Can you work these out from the model? Positions are in its coordinate system, mm. A direction names the side the tool comes from. Round coordinates to 2 decimals unless told otherwise and drop trailing zeros. Loops run counter-clockwise (first coordinate to the right, second up) from the corner with the lowest first, then second, coordinate; pieces in that order, holes last.
from build123d import *

# Parameters (mm, degrees)
F1_DEPTH = 3


with BuildPart() as f1:
    # F0 (on Front) → F1 (new body)
    with BuildSketch(Plane.XZ):
        with BuildLine():
            ThreePointArc((0, 1.75), (1.75, 0), (0, -1.75))
            Line((0, -1.75), (-0.5, -1.75))
            ThreePointArc((-0.5, -1.75), (-1.394427, -1.538854), (-2.1, -0.95))
            ThreePointArc((-2.1, -0.95), (-6.124265, -1.312868), (-4, -4.75))
            Line((-4, -4.75), (0, -4.75))
            ThreePointArc((0, -4.75), (4.75, 0), (0, 4.75))
            Line((0, 4.75), (-20, 4.75))
            ThreePointArc((-20, 4.75), (-24.75, 0), (-20, -4.75))
            Line((-20, -4.75), (-16, -4.75))
            ThreePointArc((-16, -4.75), (-13.883666, -1.297152), (-17.920914, -0.978321))
            ThreePointArc((-17.920914, -0.978321), (-18.804769, -1.662707), (-19.917848, -1.765869))
            Line((-19.917848, -1.765869), (-20, -1.75))
            ThreePointArc((-20, -1.75), (-21.75, 0), (-20, 1.75))
            Line((-20, 1.75), (0, 1.75))
        make_face()
    extrude(amount=F1_DEPTH)


solid = f1.part
(1) If we section it at A-A, the plane x = 1.25: List the corners of the cut face in (y, z) for me, then the cut area to 3 significant figures.
Worked answers:
outline: (-3, -4.58) - (0, -4.58) - (0, -1.22) - (-3, -1.22) - close; (-3, 1.22) - (0, 1.22) - (0, 4.58) - (-3, 4.58) - close
area: 20.1 mm2
(2) For faces 1 (the flat face through (-10, -3, 2)), 2 (the cylindrical face through (-21.75, -1.48, -0.04)), which set-ups out of +Z, -Z, +X, -X, +Y, -Y let a thin tool reach every point of the face, with its end or its side?
Worked answers:
face 1: +Z, -Z, +X, -X, -Y
face 2: +Y, -Y
(3) If we section it at B-B, the plane z = -3.75: List the corners of the cut face in (x, y) for me.
Worked answers:
outline: (-22.92, -3) - (-14.06, -3) - (-14.06, 0) - (-22.92, 0) - close; (-5.94, -3) - (2.92, -3) - (2.92, 0) - (-5.94, 0) - close
(4) If we section it at C-C, the plane y = -1.1: List the corners of the cut face in (x, z) for me (3 decimals), then the cut area to 3 significant figures.
Worked answers:
outline: (-20, -4.75) - (-16, -4.75) arc R2.375 ccw (long way) to (-17.921, -0.978) arc R2 cw to (-19.918, -1.766) - (-20, -1.75) arc R1.75 cw to (-20, 1.75) - (0, 1.75) arc R1.75 cw to (0, -1.75) - (-0.5, -1.75) arc R2 cw to (-2.1, -0.95) arc R2.375 ccw (long way) to (-4, -4.75) - (0, -4.75) arc R4.75 ccw to (0, 4.75) - (-20, 4.75) arc R4.75 ccw to start
area: 169 mm2
(5) If we mould it in two halves opening along Z, with no side actions, what happens to faces 3 (the flat face through (-10, -1, 4.75)), 4 (the cylindrical face through (4.75, -1.48, -0.1)), 5 (the cylindrical face through (-18.79, -1.479, -1.657)), 6 (the flat face through (-18, -1, -4.75))? For each: released by +Z, released by -Z, zero draft, split by the parting line, or undercut.
Worked answers:
face 3: released by +Z
face 4: split by the parting line
face 5: undercut
face 6: released by -Z
(6) If I drill on line 1 (Z direction, x = -10.25, y = -2.7); line 2 (X direction, y = -2.9, z = -3.75); line 3 (Z direction, x = -16.5, y = -0.9), over which ranges is the centre line in solid material (lowest first)?
Worked answers:
line 1: z = 1.75 to 4.75
line 2: x = -22.92 to -14.06, -5.94 to 2.92
line 3: z = -4.75 to -0.05, 1.75 to 4.75
(7) Will these pins go through, and if not, where does the flat tip stop? P1, Ø1, axis at y = -2, z = 3, coming from the +X side; P2, Ø0.9, axis at x = -9.5, y = -1, coming from the -Z side.
Worked answers:
P1: stops at x = 4.04
P2: stops at z = 1.75
